Can you work these out from the model? Positions are in its coordinate system, mm. A direction names the side the tool comes from. Coordinates: 2 decimals unless noted, no trailing zeros. Order: outer loops, then holes, each group sorted by start corner. A loop starts at its lowest first (then second) coordinate and runs counter-clockwise, first axis right, second up. Notation, with made-up numbers: (83.5, 79.25) -> (134.5, 79.25) arc R14 ccw to (134.5, 95.25) -> close; hole circle Ø5 at (43, 47). An arc over 180 degrees is marked (long way). Answer in a Markdown table with one row per item. Add a question column.
1. On a 3-axis mill with a long thin cutter (end or side, diameter ignored), from which of +Z, -Z, +X, -X, +Y, -Y can I reach the whole of each face in a straight line? I mean faces 1 (the face through (-1.28, 0.86, -0.51)), 2 (the face through (-1.7, 0, -1.3)). Say none if no direction works.
2. If I drill on line 1 along Y through (x, z) = (3.5, -0.05); line 2 along X through (y, z) = (0.7, -1.55), over which ranges is the centre line in solid material (lowest first)? Write a range as [from, to].
3. Imagine slicing it at B-B on x = -0.75. Write out the boundary of the cut face in (y, z), plus the area to 3 significant figures.
4. Will these pins go through, and if not, where does the flat tip stop? pin 1 (2 mm diameter, centred on x = 3.5, z = 1.5, fed in from -Y); pin 2 (0.7 mm diameter, centred on x = -1, y = 0, fed in from -Z); pin 3 (2 mm diameter, centred on x = 4, z = 0.5, fed in from +Y).
5. We'd pull the mould along Z, two halves only. Please class faces 3 (the face through (-1.28, -0.87, -0.49)), 4 (the face through (6.3, 0, 0)), 5 (the face through (3.04, -1.5, 0.07)): pulls with the +Z half, pulls with the -Z half, needs draft (parallel to the pull), parting line crosses it, or undercut.
6. Imagine slicing it at A-A on x = 4.5. Write out the boundary of the cut face in (y, z), plus the area to 3 significant figures.
Autodesk Inventor part; units mm, degrees
ref_plane "bolt_to_nut_XY" through (6.3, 0, 0) normal (1, 0, 0) x (0, 0, -1)
ref_plane "bolt_to_nut_YZ" through (6.3, 0, 0) normal (0, 0, -1) x (0, 1, 0)
ref_plane "bolt_to_nut_ZX" through (6.3, 0, 0) normal (0, 1, 0) x (1, 0, 0)
sketch "Sketch_1" plane through (0, 0, 0) normal (0, 0, 1) x (1, 0, 0)
  line L0 (6.3, 0) -> (0, 0)
  line L1 (-1.7, 0) -> (-1.7, 3)
  line L2 (-1.7, 3) -> (-1.5, 3)
  line L3 (-1.5, 3) -> (0, 1.5)
  line L4 (0, 1.5) -> (5.9935, 1.5)
  line L5 (5.9935, 1.5) -> (6.3, 1.1935)
  line L6 (6.3, 1.1935) -> (6.3, 0)
  line L7 (6.3, 0) -> (-1.7, 0)
revolve "Revolution1" add sketch "Sketch_1" angle 360 about axis through (6.3, 0, 0) along (1, 0, 0)
thread "Thread1"
sketch "Sketch2" plane through (-1.7, 0, 0) normal (-1, 0, 0) x (0, 0, 1)
  point P0 (0, 0)
hole "Hole1" at (-1.7, 0, 0) direction (1, 0, 0) diameter 2 depth 0.85 tip angle 150
sketch "Sketch_3" plane through (-1.7, 0, 0) normal (1, 0, 0) x (0, 0, -1)
  line L0 (-1, -0.5774) -> (0, -1.1547)
  line L1 (0, -1.1547) -> (1, -0.5774)
  line L2 (1, -0.5774) -> (1, 0.5774)
  line L3 (1, 0.5774) -> (0, 1.1547)
  line L4 (0, 1.1547) -> (-1, 0.5774)
  line L5 (-1, 0.5774) -> (-1, -0.5774)
extrude "Extrusion1" cut sketch "Sketch_3" along normal blind 0.85
ref_plane "bolt_to_nut_XY" through (6.3, 0, 0) normal (1, 0, 0) x (0, 0, -1)
ref_plane "bolt_to_nut_YZ" through (6.3, 0, 0) normal (0, 0, -1) x (0, 1, 0)
ref_plane "bolt_to_nut_ZX" through (6.3, 0, 0) normal (0, 1, 0) x (1, 0, 0)
ref_plane "dummy_to_bolt_XY" through (0, 0, 0) normal (1, 0, 0) x (0, 0, -1)
ref_plane "dummy_to_bolt_YZ" through (0, 0, 0) normal (0, 0, -1) x (0, 1, 0)
ref_plane "dummy_to_bolt_ZX" through (0, 0, 0) normal (0, 1, 0) x (1, 0, 0)
properties part number "HFBCM3-8"
Answers follow:
| question | item | result |
|---|---|---|
| 1 | face 1 | -X |
| 1 | face 2 | +Z, -Z, -X, +Y, -Y |
| 2 | line 1 | y = [-1.5, 1.5] |
| 2 | line 2 | x = [-1.7, -0.2] |
| 3 | outline | circle Ø4.5 at (0, 0); hole circle Ø1.25 at (0, 0) |
| 3 | area | 14.7 mm² |
| 4 | pin 1 | stops at y = -1.41 |
| 4 | pin 2 | stops at z = -2.85 |
| 4 | pin 3 | stops at y = 1.5 |
| 5 | face 3 | undercut |
| 5 | face 4 | needs draft |
| 5 | face 5 | parting line crosses it |
| 6 | outline | circle Ø3 at (0, 0) |
| 6 | area | 7.07 mm² |
